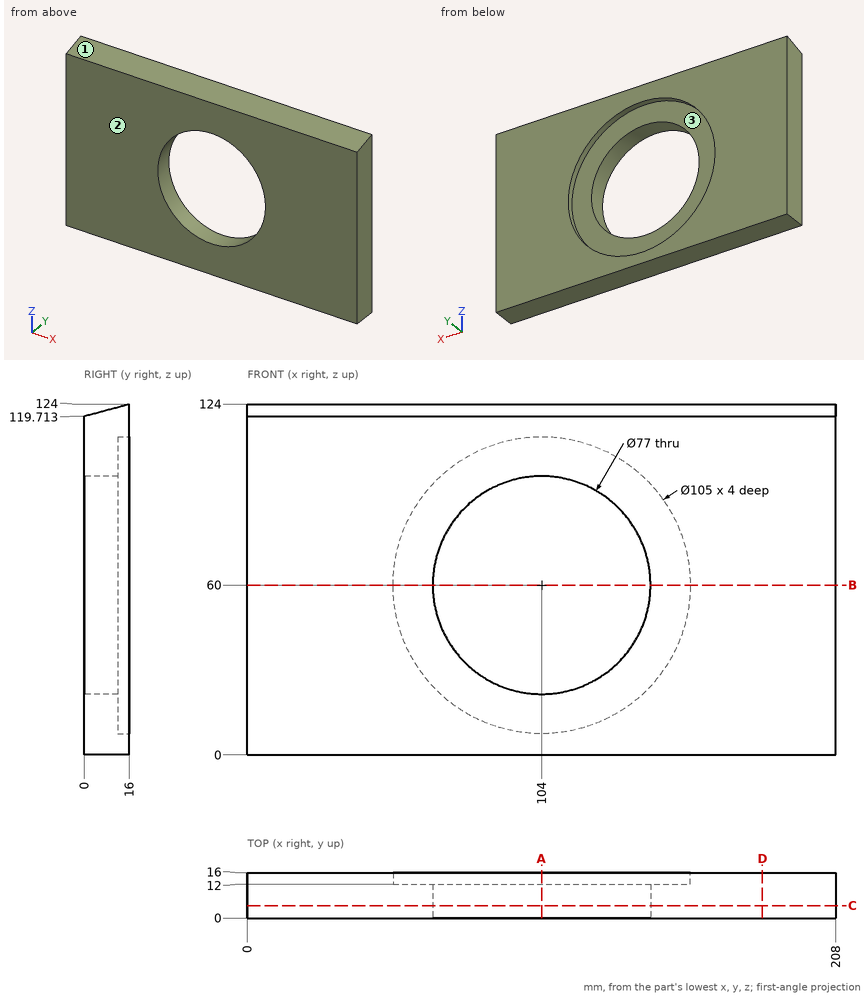
Print and shaded views of the part. All mm, measured from the part's lowest x, y and z. Coordinates: 2 decimals unless noted, no trailing zeros. Write each loop counter-clockwise with the first axis right and the second up, starting at its lowest first coordinate (ties: lowest second). Pieces come first, ordered by that corner, then holes. Notation, with made-up numbers: M 82.5,41 L 112.5,41 A13 ccw 112.5,54 Z; hole C 10,1 d1. An arc over 180 degrees is marked long. Return JSON: item names as keys, results as strings.
1. Saw through at A-A, the plane x = 104. Write the cut outline in (y, z).
Determined:
{"outline": "M 0,0 L 16,0 L 16,7.5 L 12,7.5 L 12,21.5 L 0,21.5 Z; M 0,98.5 L 12,98.5 L 12,112.5 L 16,112.5 L 16,124 L 0,119.71 Z"}
2. Probe L1, parallel to X at y = 2.25, z = 56; L2, parallel to X at y = 1.5, z = 57; L3, parallel to Z at x = 89, y = 11.25. List the from-to ranges inside material, lowest first.
Determined:
{"L1": "0 to 65.71, 142.29 to 208", "L2": "0 to 65.62, 142.38 to 208", "L3": "0 to 24.54, 95.46 to 122.73"}
3. Flat gauge pin, fed straight in: pin 1 Ø3 at (x, y) = (168.5, 12.5) entering from +Z. Where does the tip first touch, or does it go through?
Determined:
{"pin 1": "z = 123.46"}
4. Saw through at C-C, the plane y = 4.5. Write the cut outline in (x, z).
Determined:
{"outline": "M 0,0 L 208,0 L 208,120.92 L 0,120.92 Z; hole C 104,60 d77"}
5. Saw through at B-B, the plane z = 60. Write the cut outline in (x, y), then the cut area to 3 significant figures.
Determined:
{"outline": "M 0,0 L 65.5,0 L 65.5,12 L 51.5,12 L 51.5,16 L 0,16 Z; M 142.5,0 L 208,0 L 208,16 L 156.5,16 L 156.5,12 L 142.5,12 Z", "area": "1,980 mm²"}
6. Pull direction Z, two halves, no side cores. Call the marked faces 1, 2 and 3: pulls with the +Z half, pulls with the -Z half, needs draft (parallel to the pull), parting line crosses it, or undercut.
Determined:
{"face 1": "pulls with the +Z half", "face 2": "needs draft", "face 3": "undercut"}
7. Saw through at D-D, the plane x = 182. Write the cut outline in (y, z).
Determined:
{"outline": "M 0,0 L 16,0 L 16,124 L 0,119.71 Z"}
